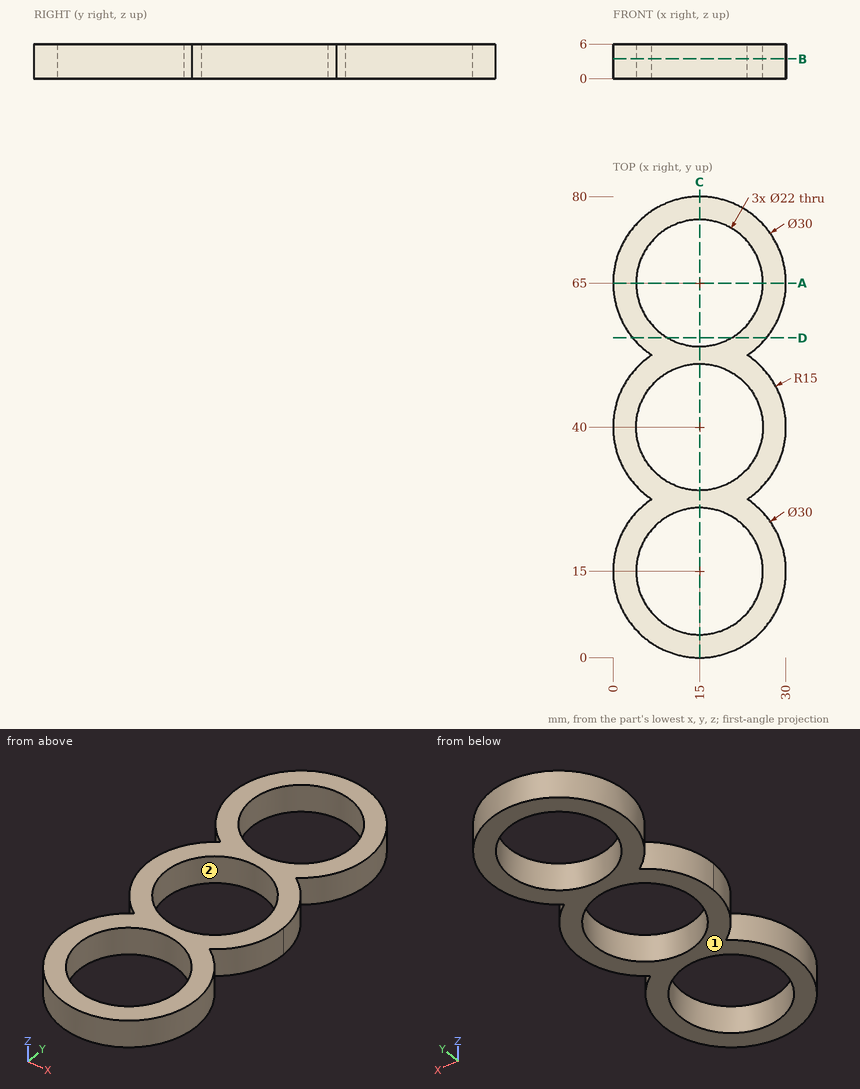
Can you work these out from the drawing? Everything is in mm from the part's minimum corner. Round coordinates to 2 decimals unless told otherwise and drop trailing zeros. Order: outer loops, then holes, each group sorted by start corner. A loop starts at its lowest first (then second) coordinate and runs counter-clockwise, first axis right, second up.
(1) If we section it at B-B (z = 3.4): Please give me the cut outline in (x, y), plus the area to 3 significant figures.
Results are:
outline: (6.71, 27.5) arc R15 ccw (long way) to (23.29, 27.5) arc R15 ccw to (23.29, 52.5) arc R15 ccw (long way) to (6.71, 52.5) arc R15 ccw to start; hole circle Ø22 at (15, 15); hole circle Ø22 at (15, 40); hole circle Ø22 at (15, 65)
area: 868 mm2
(2) If we section it at C-C (x = 15): Please give me the cut outline in (y, z).
Results are:
outline: (0, 0) - (4, 0) - (4, 6) - (0, 6) - close; (26, 0) - (29, 0) - (29, 6) - (26, 6) - close; (51, 0) - (54, 0) - (54, 6) - (51, 6) - close; (76, 0) - (80, 0) - (80, 6) - (76, 6) - close
(3) I'm going to push flat-ended pins straight in: pin 1 (1 mm diameter, centred on x = 18.5, y = 49, fed in from +Z); pin 2 (1 mm diameter, centred on x = 7.5, z = 1, fed in from -Y); pin 3 (2 mm diameter, centred on y = 29.5, z = 2.5, fed in from -X); pin 4 (2 mm diameter, centred on x = 20, z = 3, fed in from +Y). Where does each tip first touch, or does it pass through?
Results are:
pin 1: passes through
pin 2: stops at y = 1.73
pin 3: stops at x = 3.39
pin 4: stops at y = 79.46
(4) If I drill on L1, parallel to Y at x = 15, z = 4.2; L2, parallel to X at y = 40, z = 2.9; L3, parallel to Y at x = 2.5, z = 1.85, over which ranges is the centre line in solid material (lowest first)?
Results are:
L1: y = 0 to 4, 26 to 29, 51 to 54, 76 to 80
L2: x = 0 to 4, 26 to 30
L3: y = 6.71 to 23.29, 31.71 to 48.29, 56.71 to 73.29
(5) If we section it at D-D (y = 55.5): Please give me the cut outline in (x, z), plus the area to 3 significant figures.
Results are:
outline: (3.39, 0) - (9.45, 0) - (9.45, 6) - (3.39, 6) - close; (20.55, 0) - (26.61, 0) - (26.61, 6) - (20.55, 6) - close
area: 72.8 mm2
(6) If we section it at A-A (y = 65): Please give me the cut outline in (x, z).
Results are:
outline: (0, 0) - (4, 0) - (4, 6) - (0, 6) - close; (26, 0) - (30, 0) - (30, 6) - (26, 6) - close
(7) We'd pull the mould along Y, two halves only. Please class the marked faces 1 and 2: +Y half, -Y half, draft (parallel to the pull), parting line (faces both ways), or undercut.
Results are:
face 1: draft
face 2: undercut
